Check sheet for the drawn part. Datum: minimum x, y, z corner. Units: mm. A direction names the side the tool comes from. Give positions to 0.01 mm unless a question says otherwise; leave off trailing zeros. Loops run counter-clockwise (first coordinate to the right, second up) from the corner with the lowest first, then second, coordinate; pieces in that order, holes last. Notation, with made-up numbers: (24.25, 38.25) - (33.25, 38.25) arc R22 cw to (33.25, 74.25) - close; hole circle Ø3 at (-34, 67). An arc over 180 degrees is marked (long way). Answer in a Markdown table with one row per item.
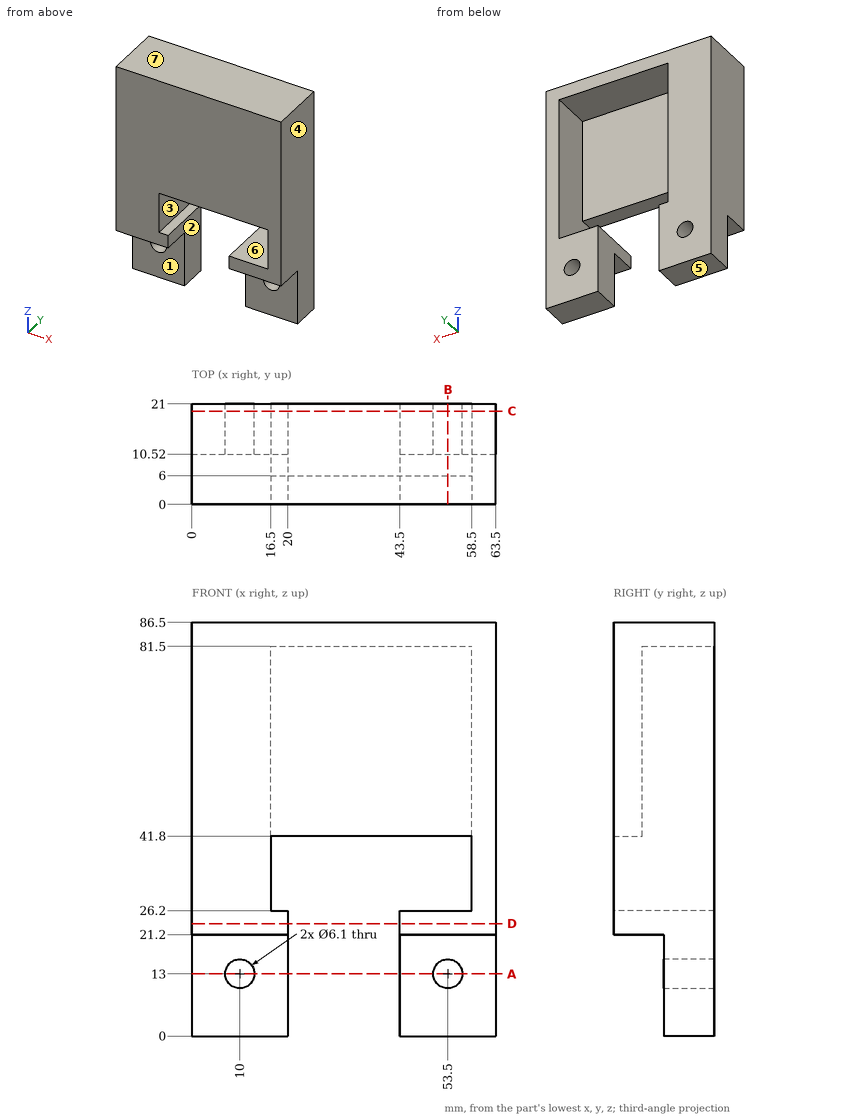
Q1. Go/stop test with flat-tipped pins: P1, Ø5.5, axis at x = 6, y = 3.5, coming from the -Z side; P2, Ø4.5, axis at x = 31.5, y = 11, coming from the -Z side; P3, Ø16, axis at x = 11, z = 12, coming from the -Y side. Record where each tip stops, or that it passes through.
Completed:
| item | result |
|---|---|
| P1 | z = 21.2 |
| P2 | z = 81.5 |
| P3 | y = 10.52 |
Q2. Sectioned sample at B-B (x = 53.5). Record the cut outline in (y, z), and give its area (3 significant figures).
Completed:
| item | result |
|---|---|
| outline | (0, 21.2) - (10.52, 21.2) - (10.52, 16.05) - (21, 16.05) - (21, 26.2) - (0, 26.2) - close; (0, 41.8) - (6, 41.8) - (6, 81.5) - (21, 81.5) - (21, 86.5) - (0, 86.5) - close; (10.52, 0) - (21, 0) - (21, 9.95) - (10.52, 9.95) - close |
| area | 606 mm^2 |
Q3. Sectioned sample at A-A (z = 13). Record the cut outline in (x, y), and give its area (3 significant figures).
Completed:
| item | result |
|---|---|
| outline | (0, 10.52) - (6.95, 10.52) - (6.95, 21) - (0, 21) - close; (13.05, 10.52) - (20, 10.52) - (20, 21) - (13.05, 21) - close; (43.5, 10.52) - (50.45, 10.52) - (50.45, 21) - (43.5, 21) - close; (56.55, 10.52) - (63.5, 10.52) - (63.5, 21) - (56.55, 21) - close |
| area | 291 mm^2 |
Q4. Sectioned sample at C-C (y = 19.5). Record the cut outline in (x, z).
Completed:
| item | result |
|---|---|
| outline | (0, 0) - (20, 0) - (20, 26.2) - (16.5, 26.2) - (16.5, 81.5) - (58.5, 81.5) - (58.5, 26.2) - (43.5, 26.2) - (43.5, 0) - (63.5, 0) - (63.5, 86.5) - (0, 86.5) - close; hole circle Ø6.1 at (10, 13); hole circle Ø6.1 at (53.5, 13) |
Q5. Tool access check on the marked faces 1, 2 and 3. Record the directions out of +Z, -Z, +X, -X, +Y, -Y that give a thin tool (end or side, any length) a straight path to the whole face; none if there is none.
Completed:
| item | result |
|---|---|
| face 1 | -Z, +X, -X, -Y |
| face 2 | -Z, +Y, -Y |
| face 3 | +Y |
Q6. Draft check along Z on the marked faces 4, 5, 6 and 7. Enter one of: +Z half, -Z half, draft (parallel to the pull), parting line (faces both ways), or undercut.
Completed:
| item | result |
|---|---|
| face 4 | draft |
| face 5 | -Z half |
| face 6 | undercut |
| face 7 | +Z half |
Q7. Sectioned sample at D-D (z = 23.5). Record the cut outline in (x, y).
Completed:
| item | result |
|---|---|
| outline | (0, 0) - (20, 0) - (20, 21) - (0, 21) - close; (43.5, 0) - (63.5, 0) - (63.5, 21) - (43.5, 21) - close |
Q8. Thickness scan on line 1 (X direction, y = 14, z = 13); line 2 (X direction, y = 8.5, z = 41); line 3 (Z direction, x = 17.5, y = 11.75). Record the ranges inside material, lowest first.
Completed:
| item | result |
|---|---|
| line 1 | 0 to 6.95, 13.05 to 20, 43.5 to 50.45, 56.55 to 63.5 |
| line 2 | 0 to 16.5, 58.5 to 63.5 |
| line 3 | 0 to 26.2, 81.5 to 86.5 |
